Part model, mm, in its own coordinate system. A direction names the side the tool comes from. Coordinates: 2 decimals unless noted, no trailing zeros. Write each loop counter-clockwise with the first axis right and the second up, starting at its lowest first coordinate (ties: lowest second). Pieces come first, ordered by that corner, then holes. Notation, with made-up numbers: (28, 4.25) -> (54, 4.25) arc R17 cw to (54, 34.25) -> close; hole circle Ø10 at (-18.5, 60). An arc over 180 degrees is marked (long way). Write item = value, one per line. Start each with the question number.
Q1. Band-saw the part on A-A, the plane x = 39.5. List the corners of the cut face in (y, z), plus the area to 3 significant figures.
Q2. Band-saw the part on D-D, the plane x = 54.5. List the corners of the cut face in (y, z).
Q3. Band-saw the part on B-B, the plane z = 0.95. List the corners of the cut face in (x, y), plus the area to 3 significant figures.
Q4. Pin check, flat tips, straight feed: P1, Ø1.5, axis at y = -42, z = 1.5, coming from the -X side; P2, Ø0.9, axis at x = 6, z = 1.5, coming from the -Y side; P3, Ø3, axis at x = 44.5, y = 20, coming from the -Z side; P4, Ø1.5, axis at y = -43, z = 2, coming from the +X side. Stop position of each tip, or through.
Q5. Probe line 1 (Y direction, x = 40, z = 0.85); line 2 (Y direction, x = 74, z = 0.8); line 3 (X direction, y = 76, z = 2.2). List the from-to ranges inside material, lowest first.
Q6. Band-saw the part on C-C, the plane y = 2.5. List the corners of the cut face in (x, z).
Q7. Pull direction Y, two halves, no side cores. Call faces 1 (the flat face through (69, -40.678, 1)), 2 (the flat face through (34.902, 76, 1)), 3 (the cylindrical face through (41.928, -0.114, 1.479)): released by +Y, released by -Y, zero draft, split by the parting line, or undercut.
Q8. Tool access for faces 4 (the flat face through (39, 20, 0)), 5 (the flat face through (10, -40.678, 1)), 6 (the flat face through (58.102, 76, 1)), 7 (the flat face through (57.121, -42, 1)), 8 (the flat face through (47.121, -42, 1)): list every direction of +Z, -Z, +X, -X, +Y, -Y with a clear straight run to the whole face (end or side of a thin tool).
from build123d import *

# Parameters (mm, degrees)
MODEL_R                 = 5
SALIENTE_EXTRUIR1_DEPTH = 3


with BuildPart() as part:
    # Model → Saliente-Extruir1 (new body)
    with BuildSketch(Plane.XY):
        Polygon((81.121222681, 81.82151488), (70.11183083, 81.82151488), (58.10243898, 81.82151488), (58.10243898, 70.02151488), (34.90243898, 70.02151488), (34.90243898, 81.82151488), (19.694696617, 81.82151488), (-1.878778155, 81.82151488), (-1.878778155, -40.67848512), (22.121222263, -40.67848512), (22.121222263, -44.17848512), (32.121222263, -44.17848512), (32.121222263, -40.67848512), (47.121222263, -40.67848512), (47.121222263, -44.17848512), (57.121222263, -44.17848512), (57.121222263, -40.67848512), (81.121222681, -40.67848512), align=None)
        with Locations((39.621222681, 4.32151488)):
            Circle(MODEL_R, mode=Mode.SUBTRACT)
    extrude(amount=SALIENTE_EXTRUIR1_DEPTH)


solid = part.part
Ans:
q1.outline = (-40.68, 0) -> (-0.68, 0) -> (-0.68, 3) -> (-40.68, 3) -> close; (9.32, 0) -> (70.02, 0) -> (70.02, 3) -> (9.32, 3) -> close
q1.area = 302 mm2
q2.outline = (-44.18, 0) -> (70.02, 0) -> (70.02, 3) -> (-44.18, 3) -> close
q3.outline = (-1.88, -40.68) -> (22.12, -40.68) -> (22.12, -44.18) -> (32.12, -44.18) -> (32.12, -40.68) -> (47.12, -40.68) -> (47.12, -44.18) -> (57.12, -44.18) -> (57.12, -40.68) -> (81.12, -40.68) -> (81.12, 81.82) -> (58.1, 81.82) -> (58.1, 70.02) -> (34.9, 70.02) -> (34.9, 81.82) -> (-1.88, 81.82) -> close; hole circle Ø10 at (39.62, 4.32)
q3.area = 9,890 mm2
q4.P1 = 22.12
q4.P2 = -40.68
q4.P3 = 0
q4.P4 = 57.12
q5.line_1 = -40.68 to -0.66, 9.31 to 70.02
q5.line_2 = -40.68 to 81.82
q5.line_3 = -1.88 to 34.9, 58.1 to 81.12
q6.outline = (-1.88, 0) -> (34.96, 0) -> (34.96, 3) -> (-1.88, 3) -> close; (44.28, 0) -> (81.12, 0) -> (81.12, 3) -> (44.28, 3) -> close
q7.face_1 = released by -Y
q7.face_2 = zero draft
q7.face_3 = undercut
q8.face_4 = -Z, +X, -X, +Y, -Y
q8.face_5 = +Z, -Z, -X, -Y
q8.face_6 = +Z, -Z, +Y
q8.face_7 = +Z, -Z, +X, -Y
q8.face_8 = +Z, -Z, -Y
